from build123d import *

# Parameters (mm, degrees)
CUT_EXTRUDE_2_DEPTH = 0.95
FILLET_1_R          = 0.1


with BuildPart() as part:
    # 草图8 → Revolve 1380 (revolve)
    with BuildSketch(Plane(origin=(0, 0, 0), x_dir=(0, 0, -1), z_dir=(1, 0, 0)), mode=Mode.PRIVATE) as revolve_1380_sk:
        with BuildLine():
            Line((0, 0), (-6.1, 0))
            ThreePointArc((-6.1, 0), (-5.919403703, 1.059811908), (-5.397999199, 2))
            Line((-5.397999199, 2), (-4.5, 2))
            Line((-4.5, 2), (-4.5, 1.1))
            Line((-4.5, 1.1), (-1.905255888, 1.1))
            Line((-1.905255888, 1.1), (0, 0))
        make_face()
    revolve(revolve_1380_sk.sketch.rotate(Axis((0, 0, 11.71), (0, 0, -1)), 90), axis=Axis((0, 0, 11.71), (0, 0, -1)))

    # 草图7 → 切除-拉伸2 (cut)
    with BuildSketch(Plane.XY.offset(6.1)):
        with BuildLine():
            Line((0.2, 0.826135582), (0.2, 0.797500009))
            ThreePointArc((0.2, 0.797500009), (0.375003701, 0.375003701), (0.797500009, 0.2))
            Line((0.797500009, 0.2), (0.826135582, 0.2))
            ThreePointArc((0.826135582, 0.2), (0.85, 0), (0.826135582, -0.2))
            Line((0.826135582, -0.2), (0.797500009, -0.2))
            ThreePointArc((0.797500009, -0.2), (0.375003701, -0.375003701), (0.2, -0.797500009))
            Line((0.2, -0.797500009), (0.2, -0.826135582))
            ThreePointArc((0.2, -0.826135582), (0, -0.85), (-0.2, -0.826135582))
            Line((-0.2, -0.826135582), (-0.2, -0.797500009))
            ThreePointArc((-0.2, -0.797500009), (-0.375003701, -0.375003701), (-0.797500009, -0.2))
            Line((-0.797500009, -0.2), (-0.826135582, -0.2))
            ThreePointArc((-0.826135582, -0.2), (-0.85, 0), (-0.826135582, 0.2))
            Line((-0.826135582, 0.2), (-0.797500009, 0.2))
            ThreePointArc((-0.797500009, 0.2), (-0.375003701, 0.375003701), (-0.2, 0.797500009))
            Line((-0.2, 0.797500009), (-0.2, 0.826135582))
            ThreePointArc((-0.2, 0.826135582), (0, 0.85), (0.2, 0.826135582))
        make_face()
    extrude(amount=-CUT_EXTRUDE_2_DEPTH, mode=Mode.SUBTRACT)

    # 圆角1
    fillet_1_edges = [part.edges().sort_by_distance(p)[0] for p in [
        (-1.1, 0, 4.5),
    ]]
    fillet(fillet_1_edges, radius=FILLET_1_R)


solid = part.part
The listing builds one solid part. Answer for the finished solid, in the listing's coordinates (mm). Give positions to 0.01 mm unless a question says otherwise; leave off trailing zeros. Write each loop counter-clockwise with the first axis right and the second up, starting at its lowest first coordinate (ties: lowest second). Pieces come first, ordered by that corner, then holes. Notation, with made-up numbers: (67.5, 33) -> (96.5, 33) arc R12 ccw to (96.5, 48) -> close; hole circle Ø1 at (21, -28). An arc over 180 degrees is marked (long way). One line per question, with ' | ' between items. Start each with the question number.
1. Section A-A (y = -1.6) is taken. Determine the outline of the cut face in (x, z).
2. For a pull along X with two mould halves and no side action, classify faces 1 (the cylindrical face through (0, 2, 5)), 2 (the flat face through (1, 1, 4.5)), 3 (the flat face through (0, 0, 5.15)) as pulls with the +X half, pulls with the -X half, needs draft (parallel to the pull), parting line crosses it, or undercut.
3. Section B-B (z = 1) is taken. Determine the outline of the cut face in (x, y), plus the area to 3 significant figures.
4. Given pin 1 Ø2 at (y, z) = (-1, 1.5) entering from -X, flat-ended and moving along its own axis, determine where the tip first touches the part or whether it passes through.
5. Section C-C (x = -1.45) is taken. Determine the outline of the cut face in (y, z), plus the area to 3 significant figures.
6. Find the intervals of material crossed by probe 1 along Y at (x, z) = (0.7, 3.5); probe 2 along X at (y, z) = (-0.4, 5.25), in increasing order.
Response values:
1) outline: (-1.2, 4.5) -> (1.2, 4.5) -> (1.2, 5.4) arc R2.77 ccw to (-1.2, 5.4) -> close
2) face 1: parting line crosses it | face 2: needs draft | face 3: undercut
3) outline: circle Ø1.15 at (0, 0) | area: 1.05 mm2
4) pin 1: x = -1.1
5) outline: (-1.38, 4.5) -> (1.38, 4.5) -> (1.38, 5.4) arc R2.85 ccw to (-1.38, 5.4) -> close | area: 3.13 mm2
6) probe 1: -0.85 to 0.85 | probe 2: -1.96 to -0.35, 0.35 to 1.96
